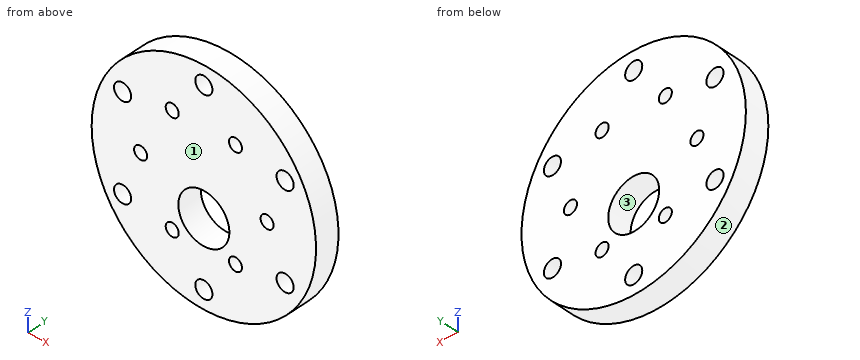
Autodesk Inventor part; units mm, degrees
ref_plane "YZ Plane" through (0, 0, 0) normal (1, 0, 0) x (0, 1, 0)
ref_plane "XZ Plane" through (0, 0, 0) normal (0, 1, 0) x (-1, 0, 0)
ref_plane "XY Plane" through (0, 0, 0) normal (0, 0, 1) x (1, 0, 0)
sketch "Sketch1" plane through (0, 0, 0) normal (0, 1, 0) x (-1, 0, 0)
  circle A0 centre (0, 0) radius 27.5
  circle A1 centre (0, -7) radius 6.25
  circle A2 centre (15.5, 0) radius 1.6
  circle A3 centre (7.75, 13.4234) radius 1.6
  circle A4 centre (-7.75, 13.4234) radius 1.6
  circle A5 centre (-15.5, 0) radius 1.6
  circle A6 centre (-7.75, -13.4234) radius 1.6
  circle A7 centre (7.75, -13.4234) radius 1.6
  circle A8 centre (0, 23) radius 2.1
  circle A9 centre (-19.9186, 11.5) radius 2.1
  circle A10 centre (-19.9186, -11.5) radius 2.1
  circle A11 centre (0, -23) radius 2.1
  circle A12 centre (19.9186, -11.5) radius 2.1
  circle A13 centre (19.9186, 11.5) radius 2.1
  dimension "d0" = 55
  dimension "d1" = 12.5
  dimension "d2" = 7
  dimension "d3" = 3.2
  dimension "d4" = 15.5
  dimension "d7" = 360
  dimension "d9" = 4.2
  dimension "d10" = 23
  dimension "d13" = 360
extrude "Extrusion1" add sketch "Sketch1" along normal blind 6
properties part number "motor_mounting_plate"
Can you work these out from the model? Positions are in its coordinate system, mm. Face numbers are marked on the shaded views. Coordinates: 2 decimals unless noted, no trailing zeros. Order: outer loops, then holes, each group sorted by start corner. A loop starts at its lowest first (then second) coordinate and runs counter-clockwise, first axis right, second up. Notation, with made-up numbers: (-6, 12.25) -> (26, 12.25) arc R34 cw to (26, 48.25) -> close; hole circle Ø1 at (25, 18.25). An arc over 180 degrees is marked (long way). Write each question's results on one line, items separated by ' | '.
Item 1: I want a section at C-C, the plane z = -7. Write out the boundary of the cut face in (x, y).
Results are:
outline: (-26.59, 0) -> (-6.25, 0) -> (-6.25, 6) -> (-26.59, 6) -> close; (6.25, 0) -> (26.59, 0) -> (26.59, 6) -> (6.25, 6) -> close
Item 2: I want a section at B-B, the plane x = 15.5. Write out the boundary of the cut face in (y, z).
Results are:
outline: (0, -22.72) -> (6, -22.72) -> (6, -1.6) -> (0, -1.6) -> close; (0, 1.6) -> (6, 1.6) -> (6, 22.72) -> (0, 22.72) -> close
Item 3: I want a section at D-D, the plane y = 5.05. Count the separate pieces of the cut face and the enclosed holes in it, then the cut area to 3 significant figures.
Results are:
separate pieces: 1 | enclosed holes: 13 | area: 2,120 mm²
Item 4: I'm going to push flat-ended pins straight in: pin 1 Ø4 at (x, z) = (-15.5, 0) entering from +Y; pin 2 Ø3 at (x, z) = (-7.75, -13.42) entering from -Y; pin 3 Ø1 at (x, y) = (17.5, 2.5) entering from -Z; pin 4 Ø3 at (x, y) = (14, 2) entering from +Z. Where does each tip first touch, or does it pass through?
Results are:
pin 1: y = 6 | pin 2: through | pin 3: z = -21.62 | pin 4: z = 24.49
Item 5: If I drill on line 1 along Z through (x, y) = (0, 5.75); line 2 along Z through (x, y) = (18, 4.8); line 3 along Z through (x, y) = (-1, 2.3), over which ranges is the centre line in solid material (lowest first)?
Results are:
line 1: -27.5 to -25.1, -20.9 to -13.25, -0.75 to 20.9, 25.1 to 27.5 | line 2: -20.79 to -12.35, -10.65 to 10.65, 12.35 to 20.79 | line 3: -27.48 to -24.85, -21.15 to -13.17, -0.83 to 21.15, 24.85 to 27.48
Item 6: If we mould it in two halves opening along X, with no side actions, what happens to the marked faces 1, 2 and 3? For each: +X half, -X half, draft (parallel to the pull), parting line (faces both ways), or undercut.
Results are:
face 1: draft | face 2: parting line | face 3: undercut
Item 7: I want a section at A-A, the plane x = 0. Write out the boundary of the cut face in (y, z), then the cut area to 3 significant figures.
Results are:
outline: (0, -27.5) -> (6, -27.5) -> (6, -25.1) -> (0, -25.1) -> close; (0, -20.9) -> (6, -20.9) -> (6, -13.25) -> (0, -13.25) -> close; (0, -0.75) -> (6, -0.75) -> (6, 20.9) -> (0, 20.9) -> close; (0, 25.1) -> (6, 25.1) -> (6, 27.5) -> (0, 27.5) -> close | area: 205 mm²
